Geometry check sheet. Reference: the model listing, model coordinates, mm. Give positions to 0.01 mm unless a question says otherwise; leave off trailing zeros. Order: outer loops, then holes, each group sorted by start corner. A loop starts at its lowest first (then second) coordinate and runs counter-clockwise, first axis right, second up.
from build123d import *

# Parameters (mm, degrees)
PAD_DEPTH    = 120
SKETCH001_W  = 106.691582
SKETCH001_H  = 157.654909
POCKET_DEPTH = 17.1595098612


with BuildPart() as part:
    # Sketch → Pad (new body)
    with BuildSketch(Plane.XZ):
        with BuildLine():
            ThreePointArc((35, -12), (18.5, -3.0833333333), (0, 0))
            Line((0, 0), (0, -4))
            ThreePointArc((32.5456537619, -15.1585098612), (17.2027027027, -6.8671171171), (0, -4))
            Line((32.5456537619, -15.1585098612), (35, -12))
        make_face()
    extrude(amount=PAD_DEPTH)

    # Sketch001 (on DatumPlane) → Pocket (cut, through all)
    with BuildSketch(Plane.XY.offset(2)):
        with Locations((20.474781, -55.6624445)):
            Rectangle(SKETCH001_W, SKETCH001_H)
        with BuildLine():
            ThreePointArc((32.2524687129, -7.8526368005), (29.5296070486, -0.7946159813), (22.0631189103, -2.0116568221))
            ThreePointArc((22.0631189103, -2.0116568221), (5.7021367812, -28.9781159479), (0, -60))
            ThreePointArc((0, -60), (5.7021367812, -91.0218840521), (22.0631189103, -117.9883431779))
            ThreePointArc((22.0631189103, -117.9883431779), (29.5296070486, -119.2053840187), (32.2524687129, -112.1473631995))
            ThreePointArc((24, -60), (26.075875076, -86.3981567942), (32.2524687129, -112.1473631995))
            ThreePointArc((32.2524687129, -7.8526368005), (26.075875076, -33.6018432058), (24, -60))
        make_face(mode=Mode.SUBTRACT)
        with BuildLine():
            ThreePointArc((25.051475478, -115.329447726), (27.5403048575, -115.7351280062), (28.4479254122, -113.3824543998))
            ThreePointArc((20, -60), (22.1250414169, -87.0233874705), (28.4479254122, -113.3824543998))
            ThreePointArc((28.4479254122, -6.6175456002), (22.1250414169, -32.9766125295), (20, -60))
            ThreePointArc((28.4479254122, -6.6175456002), (27.5403048575, -4.2648719938), (25.051475478, -4.670552274))
            ThreePointArc((25.051475478, -4.670552274), (9.4406810347, -30.4005388332), (4, -60))
            ThreePointArc((4, -60), (9.4406810347, -89.5994611668), (25.051475478, -115.329447726))
        make_face()
    extrude(amount=-POCKET_DEPTH, mode=Mode.SUBTRACT)


solid = part.part
Item 1: Sectioned sample at C-C (z = -13.5). Enter the section's corners in (x, y), and give its area (3 significant figures).
Reported:
outline: (30.29, -118.69) arc R6 ccw to (32.25, -112.15) arc R168.89 cw to (30.29, -105.67) - close; (30.29, -14.33) arc R168.89 cw to (32.25, -7.85) arc R6 ccw to (30.29, -1.31) - close
area: 35.1 mm2
Item 2: Sectioned sample at A-A (x = 14). Enter the section's corners in (y, z).
Reported:
outline: (-107.4, -5.88) - (-99.56, -5.88) - (-99.56, -1.74) - (-107.4, -1.74) - close; (-20.44, -5.88) - (-12.6, -5.88) - (-12.6, -1.74) - (-20.44, -1.74) - close
Item 3: Sectioned sample at D-D (z = -1.25). Enter the section's corners in (x, y), and give its area (3 significant figures).
Reported:
outline: (11.88, -103.94) - (11.88, -95.34) arc R83.24 cw to (11.88, -24.66) - (11.88, -16.06) arc R87.24 ccw to start
area: 331 mm2
Item 4: Gauge pin test, flat ends, axial feed: pin 1 (6 mm diameter, centred on x = 7, y = -56.5, fed in from +Z); pin 2 (8 mm diameter, centred on x = 19, z = -2.5, fed in from -Y); pin 3 (8 mm diameter, centred on x = 8.5, z = -2, fed in from +Y). Record the tip position at first contact, or that the pin passes through.
Reported:
pin 1: stops at z = -0.14
pin 2: stops at y = -118.35
pin 3: stops at y = -15
Item 5: Sectioned sample at B-B (y = -82). Enter the section's corners in (x, z) (3 decimals), and give its area (3 significant figures).
Reported:
outline: (2.82, -4.075) arc R53.042 cw to (6.96, -4.459) - (6.96, -0.426) arc R57.042 ccw to (2.82, -0.07) - close; (21.405, -8.511) arc R53.042 cw to (25.439, -10.498) - (25.439, -5.987) arc R57.042 ccw to (21.405, -4.169) - close
area: 34.5 mm2
Item 6: Scan lines: L1, parallel to X at y = -114, z = -10.75; L2, parallel to Y at x = 16.5, z = -4.75; L3, parallel to Y at x = 11, z = -3. Record each from-to range of solid material in increasing order.
Reported:
L1: x = 28.55 to 32.55
L2: y = -111.05 to -103.87, -16.13 to -8.95
L3: y = -102.41 to -93.41, -26.59 to -17.59
